```python
from build123d import *

# Parameters (mm, degrees)
F0_R     = 4
F1_DEPTH = 8
F2_R     = 3.0338863289
F3_DEPTH = 9.4
F4_R     = 6.3699570271
F5_DEPTH = 1
F6_R     = 1


# Not quite as in the source:
# - a fillet or chamfer that OpenCascade refuses, or shapes differently, is made with other operations: its cross-section is extruded or revolved along the edge and cut away or added


with BuildPart() as f1:
    # F0 (on Top) → F1 (new body)
    with BuildSketch(Plane.XY):
        Circle(F0_R)
    extrude(amount=F1_DEPTH)

    # F2 (on Top) → F3 (cut)
    with BuildSketch(Plane.XY):
        Circle(F2_R)
    extrude(amount=F3_DEPTH, mode=Mode.SUBTRACT)

    # F4 (on Top) → F5 (join)
    with BuildSketch(Plane.XY):
        Circle(F4_R)
    extrude(amount=F5_DEPTH)

    # F6
    f6_edges = [f1.edges().sort_by_distance(p)[0] for p in [
        (-4, 0, 1),
    ]]
    fillet(f6_edges, radius=F6_R)

    # F7: fillet of radius 1 on 2 edges, made by hand

    # F7_s1 → F7_t2 (revolve, cut)
    with BuildSketch(Plane.XZ):
        with BuildLine():
            ThreePointArc((6.3699570271, 1), (6.0770638082, 0.2928932188), (5.3699570271, 0))
            Line((5.3699570271, 0), (6.3699570271, 0))
            Line((6.3699570271, 0), (6.3699570271, 1))
        make_face()
    revolve(axis=Axis((0, 0, 0), (0, 0, 1)), mode=Mode.SUBTRACT)

    # F7_s3 → F7_t4 (revolve, cut)
    with BuildSketch(Plane.XZ):
        with BuildLine():
            ThreePointArc((4, 7), (3.7071067812, 7.7071067812), (3, 8))
            Line((3, 8), (4, 8))
            Line((4, 8), (4, 7))
        make_face()
    revolve(axis=Axis((0, 0, 8), (0, 0, 1)), mode=Mode.SUBTRACT)


solid = f1.part
```
The listing builds one solid part. Answer for the finished solid, in the listing's coordinates (mm). Give positions to 0.01 mm unless a question says otherwise; leave off trailing zeros. Write each loop counter-clockwise with the first axis right and the second up, starting at its lowest first coordinate (ties: lowest second). Pieces come first, ordered by that corner, then holes. Notation, with made-up numbers: (21, -38) -> (58, -38) arc R17 cw to (58, -24) -> close; hole circle Ø8 at (-30, 9). An arc over 180 degrees is marked (long way). Write item = value, one per line. Start each with the question number.
1) The part is cut by section A-A, the plane x = 0. Determine the outline of the cut face in (y, z), and give its area (3 significant figures).
2) The part is cut by section C-C, the plane z = 6. Determine the outline of the cut face in (x, y), and give its area (3 significant figures).
3) Determine the mould class of faces 1 (the face through (0, 0, 0)), 2 (the face through (-2.236, 2.05, 4.451)), 3 (the face through (-0.867, -3.905, 4.465)) for opening direction X: +X half, -X half, draft (parallel to the pull), parting line (faces both ways), or undercut.
4) The part is cut by section D-D, the plane z = 1.5. Determine the outline of the cut face in (x, y), and give its area (3 significant figures).
5) Straight lines are drawn through the part: line 1 along Y through (x, z) = (0, 2.75); line 2 along Z through (x, y) = (1, 1). For each, find the intervals that lie inside material, in ascending order.
6) Each of these flat-tipped pins is pushed along its axis until it touches: pin 1 (3.5 mm diameter, centred on x = 0, y = 0, fed in from +Z); pin 2 (2 mm diameter, centred on x = -2, z = 3.5, fed in from -Y); pin 3 (1 mm diameter, centred on y = 4, z = 2.5, fed in from +X). Where does it stop, or does it pass through?
Solutions:
q1.outline = (-6.37, 1) arc R1 ccw to (-5.37, 0) -> (5.37, 0) arc R1 ccw to (6.37, 1) -> (5, 1) arc R1 cw to (4, 2) -> (4, 7) arc R1 ccw to (3.03, 8) -> (3.03, 1) -> (-3.03, 1) -> (-3.03, 8) arc R1 ccw to (-4, 7) -> (-4, 2) arc R1 cw to (-5, 1) -> close
q1.area = 25.8 mm²
q2.outline = circle Ø8 at (0, 0); hole circle Ø6.07 at (0, 0)
q2.area = 21.3 mm²
q3.face_1 = draft
q3.face_2 = undercut
q3.face_3 = parting line
q4.outline = circle Ø8.27 at (0, 0); hole circle Ø6.07 at (0, 0)
q4.area = 24.8 mm²
q5.line_1 = -4 to -3.03, 3.03 to 4
q5.line_2 = 0 to 1
q6.pin_1 = 1
q6.pin_2 = -3.87
q6.pin_3 = 1.94
